```python
from build123d import *

# Parameters (mm, degrees)
F0_W     = 50
F0_H     = 50
F0_W_2   = 46
F0_H_2   = 46
F1_DEPTH = 1100
F2_R     = 12
F3_DEPTH = 50.001
F4_R     = 10
F5_DEPTH = 50.001
F6_R     = 10
F6_R_2   = 4
F7_DEPTH = 2


with BuildPart() as f1:
    # F0 (on Front) → F1 (new body)
    with BuildSketch(Plane.XZ):
        with Locations((25, 25)):
            Rectangle(F0_W, F0_H)
        with Locations((25, 25)):
            Rectangle(F0_W_2, F0_H_2, mode=Mode.SUBTRACT)
    extrude(amount=F1_DEPTH)

    # F2 (on face) → F3 (cut, through all)
    with BuildSketch(Plane.XY.offset(50)):
        with Locations((25, -500)):
            Circle(F2_R)
        with Locations((25, -240)):
            Circle(F2_R)
    extrude(amount=-F3_DEPTH, mode=Mode.SUBTRACT)

    # F4 (on face) → F5 (cut, through all)
    with BuildSketch(Plane.XY.offset(50)):
        with Locations((25, -840)):
            Circle(F4_R)
    extrude(amount=-F5_DEPTH, mode=Mode.SUBTRACT)

    # F6 (on face) → F7 (join)
    with BuildSketch(Plane.XY.offset(50)):
        with Locations((25, -840)):
            Circle(F6_R)
        with Locations((25, -840)):
            Circle(F6_R_2, mode=Mode.SUBTRACT)
    extrude(amount=-F7_DEPTH)


solid = f1.part
```
Could you check a few things on this model? Use its own coordinates, in mm. A direction names the side the tool comes from. Coordinates: 2 decimals unless noted, no trailing zeros. Write each loop counter-clockwise with the first axis right and the second up, starting at its lowest first coordinate (ties: lowest second). Pieces come first, ordered by that corner, then holes. Notation, with made-up numbers: (-38.5, 44.25) - (18.5, 44.25) arc R20 cw to (18.5, 66.25) - close; hole circle Ø6 at (16, -11.75). An arc over 180 degrees is marked (long way). Use a Markdown table: item, result.
Q1. Please list where these lines run through material, in increasing order: L1, parallel to Y at x = 25, z = 1.45; L2, parallel to Y at x = 25, z = 49.5; L3, parallel to Z at x = 32.5, y = -661.
Geometry check:
| item | result |
|---|---|
| L1 | y = -1100 to -850, -830 to -512, -488 to -252, -228 to 0 |
| L2 | y = -1100 to -844, -836 to -512, -488 to -252, -228 to 0 |
| L3 | z = 0 to 2, 48 to 50 |
Q2. Thinking about a two-plate mould opening in X: for faces 4 (the flat face through (0, -542, 25)), 5 (the flat face through (25, -542, 0)), 6 (the cylindrical face through (23.44, -228.1, 1.01)), which applies, +X half, -X half, draft (parallel to the pull), parting line (faces both ways), or undercut?
Geometry check:
| item | result |
|---|---|
| face 4 | -X half |
| face 5 | draft |
| face 6 | undercut |
Q3. Imagine slicing it at A-A (y = -500). List the corners of the cut face in (x, z) for me, and give its area (3 significant figures).
Geometry check:
| item | result |
|---|---|
| outline | (0, 0) - (13, 0) - (13, 2) - (2, 2) - (2, 48) - (13, 48) - (13, 50) - (0, 50) - close; (37, 0) - (50, 0) - (50, 50) - (37, 50) - (37, 48) - (48, 48) - (48, 2) - (37, 2) - close |
| area | 288 mm2 |
Q4. Which directions (+Z, -Z, +X, -X, +Y, -Y) give clear straight access to the entire face, cutting with the end or side of a thin tool? Please do faces 1 (the flat face through (2, -542, 25)), 2 (the cylindrical face through (23.44, -488.1, 1.01)), 3 (the cylindrical face through (23.698, -830.085, 1.014)).
Geometry check:
| item | result |
|---|---|
| face 1 | +Y, -Y |
| face 2 | +Z, -Z |
| face 3 | -Z |
Q5. Imagine slicing it at B-B (z = 40.5). List the corners of the cut face in (x, y) for me.
Geometry check:
| item | result |
|---|---|
| outline | (0, -1100) - (2, -1100) - (2, 0) - (0, 0) - close; (48, -1100) - (50, -1100) - (50, 0) - (48, 0) - close |
Q6. Imagine slicing it at C-C (y = -361). List the corners of the cut face in (x, z) for me.
Geometry check:
| item | result |
|---|---|
| outline | (0, 0) - (50, 0) - (50, 50) - (0, 50) - close; hole (2, 2) - (48, 2) - (48, 48) - (2, 48) - close |
